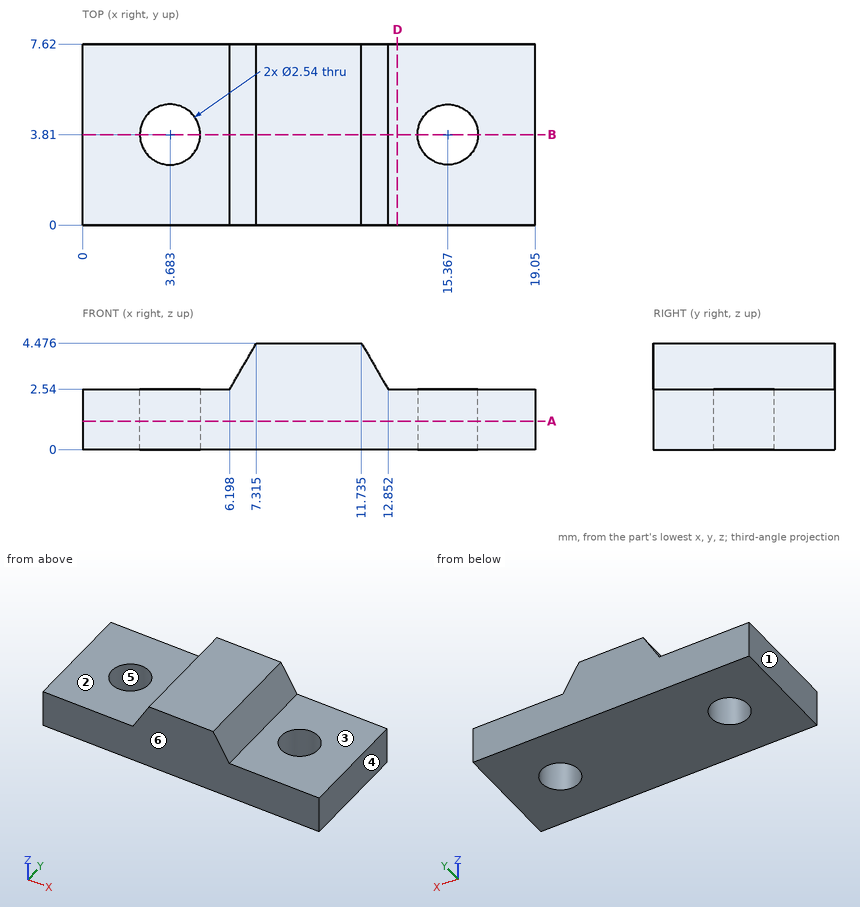
Study the drawing (mm; zero at the part's minimum x, y, z) and answer. A direction names the side the tool comes from. Give positions to 0.01 mm unless a question says otherwise; leave off trailing zeros. Order: outer loops, then holes, each group sorted by start corner. A loop starts at its lowest first (then second) coordinate and runs counter-clockwise, first axis right, second up. Notation, with made-up numbers: (62.25, 21.25) - (120.25, 21.25) arc R22 ccw to (120.25, 46.25) - close; hole circle Ø2 at (8.5, 68.5). An arc over 180 degrees is marked (long way). Answer as CSV lines item,"result". Start each with the question number.
Q1. The part is cut by section B-B (y = 3.81). Give the number of separate pieces and of enclosed holes in the cut face, then the cut area to 3 significant figures.
Q2. The part is cut by section D-D (x = 13.25). Write down the section's boundary in (y, z).
Q3. Given pin 1 Ø3 at (x, y) = (4, 3) entering from +Z; pin 2 Ø2 at (y, z) = (2, 3.5) entering from -X, each flat-ended and moving along its own axis, determine where each tip first touches the part or whether it passes through.
Q4. The part is cut by section A-A (z = 1.2). Write down the section's boundary in (x, y), then the cut area to 3 significant figures.
Q5. The mould has two halves that part along Y. Classify the marked faces 4, 5 and 6: +Y half, -Y half, draft (parallel to the pull), parting line (faces both ways), or undercut.
Q6. Find the intervals of material crossed by L1, parallel to Z at x = 14.25, y = 5.75; L2, parallel to Z at x = 6.5, y = 2.75 (1 decimal); L3, parallel to X at y = 3.25, z = 3.85 (1 decimal), in increasing order. Write a range as [from, to].
Q7. For the marked faces 1, 2 and 3, determine the directions among +Z, -Z, +X, -X, +Y, -Y from which every point of the face is accessible in a straight line to the end or side of a thin tool.
Check result:
1,separate pieces,"3"
1,enclosed holes,"0"
1,area,"46.2 mm²"
2,outline,"(0, 0) - (7.62, 0) - (7.62, 2.54) - (0, 2.54) - close"
3,pin 1,"stops at z = 2.54"
3,pin 2,"stops at x = 0"
4,outline,"(0, 0) - (19.05, 0) - (19.05, 7.62) - (0, 7.62) - close; hole circle Ø2.54 at (3.68, 3.81); hole circle Ø2.54 at (15.37, 3.81)"
4,area,"135 mm²"
5,face 4,"draft"
5,face 5,"undercut"
5,face 6,"-Y half"
6,L1,"z = [0, 2.54]"
6,L2,"z = [0, 3.1]"
6,L3,"x = [7, 12.1]"
7,face 1,"+Z, -Z, -X, +Y, -Y"
7,face 2,"+Z, -X, +Y, -Y"
7,face 3,"+Z, +X, +Y, -Y"
